Read the model definition and answer for the solid it produces. Units are mm, in the model's axes. Face numbers are marked on the shaded views. A direction names the side the tool comes from. Coordinates: 2 decimals unless noted, no trailing zeros. Write each question's results on one line, items separated by ' | '.
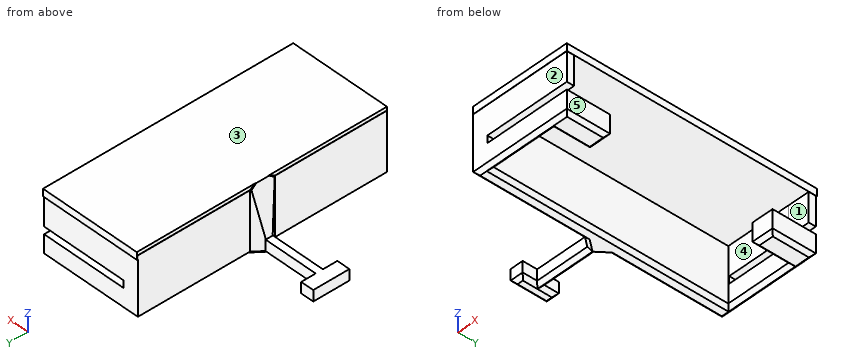
```python
from build123d import *

# Parameters (mm, degrees)
F1_DEPTH  = 18
F2_SIZE   = 0.99999
F4_W      = 49.3712280877
F4_H      = 16.5352197364
F6_W      = 25.0472677872
F6_H      = 14.5927555859
F8_W      = 28.0247684568
F8_H      = 69.3199932575
F9_DEPTH  = 2
F11_W     = 7.2507392615
F11_H     = 64.9974308908
F12_DEPTH = 10
F13_W     = 37.7304842696
F13_H     = 75.3901228309
F14_DEPTH = 2


# Not quite as in the source:
# - a fillet or chamfer is up to 0.001 mm smaller than in the source, because OpenCascade refuses the exact size


with BuildPart() as f1:
    # F0 (on Top) → F1 (new body)
    with BuildSketch(Plane.XY):
        Polygon((-8.5048572017, 5), (-12.1048572017, 5), (-12.1048572017, 0), (-12.1048572017, -5), (-8.5048572017, -5), (-8.5048572017, -1), (6.4951427983, -1), (8.4951427983, -3.4849380649), (8.4951427983, -34.5), (36.4951427983, -34.5), (36.4951427983, -22.5), (30.4951427983, -22.5), (30.4951427983, -32.5), (12.4951427983, -32.5), (12.4951427983, 0), (12.4951427983, 32.5), (30.4951427983, 32.5), (30.4951427983, 22.5), (36.4951427983, 22.5), (36.4951427983, 34.5), (8.4951427983, 34.5), (8.4951427983, 3.4849380649), (6.4951427983, 1), (-8.5048572017, 1), align=None)
    extrude(amount=F1_DEPTH)

    # F2 (size 1 in the source; OpenCascade refuses exactly that, so slightly less here)
    f2_edges = [f1.edges().sort_by_distance(p)[0] for p in [
        (-10.304857, 5, 18),
        (-12.104857, 0, 18),
        (-10.304857, -5, 18),
        (-8.504857, -3, 18),
        (-1.004857, -1, 18),
        (7.495143, -2.242469, 18),
        (8.495143, -18.992469, 18),
        (22.495143, -34.5, 18),
        (36.495143, -28.5, 18),
        (33.495143, -22.5, 18),
        (30.495143, -27.5, 18),
        (21.495143, -32.5, 18),
        (12.495143, 0, 18),
        (21.495143, 32.5, 18),
        (30.495143, 27.5, 18),
        (33.495143, 22.5, 18),
        (36.495143, 28.5, 18),
        (22.495143, 34.5, 18),
        (8.495143, 18.992469, 18),
        (7.495143, 2.242469, 18),
        (-1.004857, 1, 18),
        (-8.504857, 3, 18),
        (-10.304857, 5, 0),
        (-12.104857, 0, 0),
        (-10.304857, -5, 0),
        (-8.504857, -3, 0),
        (-1.004857, -1, 0),
        (7.495143, -2.242469, 0),
        (8.495143, -18.992469, 0),
        (22.495143, -34.5, 0),
        (36.495143, -28.5, 0),
        (33.495143, -22.5, 0),
        (30.495143, -27.5, 0),
        (21.495143, -32.5, 0),
        (12.495143, 0, 0),
        (21.495143, 32.5, 0),
        (30.495143, 27.5, 0),
        (33.495143, 22.5, 0),
        (36.495143, 28.5, 0),
        (22.495143, 34.5, 0),
        (8.495143, 18.992469, 0),
        (7.495143, 2.242469, 0),
        (-1.004857, 1, 0),
        (-8.504857, 3, 0),
    ]]
    chamfer(f2_edges, length=F2_SIZE)

    # F4 (on offset) → F7 section 0
    with BuildSketch(Plane.XY.offset(4)):
        with Locations((-18.2442103978, -0.0910270028)):
            Rectangle(F4_W, F4_H)
    # F6 (on offset) → F7 section 1
    with BuildSketch(Plane.XY.offset(18)):
        with Locations((-4.1036796756, 0.1169494353)):
            Rectangle(F6_W, F6_H)
    loft(mode=Mode.SUBTRACT)

    # F8 (on offset) → F9 (join)
    with BuildSketch(Plane.XY.offset(18)):
        with Locations((22.5351126865, 0.1127310097)):
            Rectangle(F8_W, F8_H)
    extrude(amount=-F9_DEPTH)

    # F11 (on offset) → F12 (cut)
    with BuildSketch(Plane.XY.offset(6)):
        with Locations((34.090702422, 0.0231582671)):
            Rectangle(F11_W, F11_H)
    extrude(amount=F12_DEPTH, mode=Mode.SUBTRACT)

    # F13 (on offset) → F14 (cut)
    with BuildSketch(Plane.XY.offset(6)):
        with Locations((31.6290971823, -0.1884736121)):
            Rectangle(F13_W, F13_H)
    extrude(amount=F14_DEPTH, mode=Mode.SUBTRACT)


solid = f1.part
```
(1) Straight lines are drawn through the part: line 1 (Y direction, x = 28.5, z = 11.5); line 2 (X direction, y = 23.5, z = 4.5); line 3 (Z direction, x = 25, y = -12.5). For each, find the intervals that lie inside material, in ascending order.
Conclusion:
line 1: -34.5 to -32.5, 32.5 to 34.5 | line 2: 8.5 to 12.5, 30.5 to 36.5 | line 3: 16 to 18
(2) The mould has two halves that part along Y. Classify the marked faces 1, 2 and 3: pulls with the +Y half, pulls with the -Y half, needs draft (parallel to the pull), parting line crosses it, or undercut.
Conclusion:
face 1: undercut | face 2: pulls with the -Y half | face 3: needs draft
(3) Given pin 1 (8 mm diameter, centred on x = -2, y = 2, fed in from +Z); pin 2 (1.5 mm diameter, centred on x = -10, z = 3, fed in from +Y); pin 3 (5 mm diameter, centred on x = 29, y = 16.5, fed in from -Z); pin 4 (3 mm diameter, centred on x = 6, y = 3, fed in from +Z), each flat-ended and moving along its own axis, determine where each tip first touches the part or whether it passes through.
Conclusion:
pin 1: z = 4 | pin 2: y = 5 | pin 3: z = 16 | pin 4: through
(4) For the marked faces 4 and 5, determine the directions among +Z, -Z, +X, -X, +Y, -Y from which every point of the face is accessible in a straight line to the end or side of a thin tool.
Conclusion:
face 4: -Z | face 5: -Z, +X, +Y, -Y
